from build123d import *

# Parameters (mm, degrees)
SKETCH1_R                    = 18.4
BOSS_EXTRUDE1_DEPTH          = 26.5
SKETCH2_R                    = 17.4
BOSS_EXTRUDE2_DEPTH          = 31
SKETCH3_R                    = 6
BOSS_EXTRUDE3_DEPTH          = 6.5
FILLET1_R                    = 0.5
SKETCH4_R                    = 3
BOSS_EXTRUDE4_DEPTH          = 15.5
CUT_EXTRUDE1_START           = -12
CUT_EXTRUDE1_DEPTH           = 12
F_3_0_3_DIAMETER_HOLE1_D     = 3
F_3_0_3_DIAMETER_HOLE1_DEPTH = 3
F_3_0_3_DIAMETER_HOLE1_TIP   = 0.901290929
CUT_EXTRUDE2_DEPTH           = 1
SKETCH9_R                    = 4
BOSS_EXTRUDE5_DEPTH          = 1
FILLET2_R                    = 0.5
SKETCH10_R                   = 14
BOSS_EXTRUDE6_DEPTH          = 1.5
SKETCH11_W                   = 3.5
SKETCH11_H                   = 1
BOSS_EXTRUDE7_DEPTH          = 5.6
FILLET3_R                    = 0.5
SKETCH13_R                   = 9
BOSS_EXTRUDE8_DEPTH          = 3
SKETCH14_R                   = 1.5
BOSS_EXTRUDE9_DEPTH          = 8.55
FILLET4_R                    = 0.5
SKETCH15_R                   = 16.4
BOSS_EXTRUDE10_DEPTH         = 15.26


with BuildPart() as part:
    # Sketch1 → Boss-Extrude1 (new body)
    with BuildSketch(Plane.XY):
        Circle(SKETCH1_R)
    extrude(amount=BOSS_EXTRUDE1_DEPTH)

    # Sketch2 → Boss-Extrude2 (add)
    with BuildSketch(Plane(origin=(0, 0, 0), x_dir=(-1, 0, 0), z_dir=(0, 0, -1))):
        with Locations(Location((0, 0, 0), (0, 0, 180))):
            Circle(SKETCH2_R)
    extrude(amount=BOSS_EXTRUDE2_DEPTH)

    # Sketch3 → Boss-Extrude3 (add)
    with BuildSketch(Plane.XY.offset(26.5)):
        with Locations(Location((7, 0, 0), (0, 0, 180))):
            Circle(SKETCH3_R)
    extrude(amount=BOSS_EXTRUDE3_DEPTH)

    # Fillet1
    fillet1_edges = [part.edges().sort_by_distance(p)[0] for p in [
        (13, 0, 33),
    ]]
    fillet(fillet1_edges, radius=FILLET1_R)

    # Sketch4 → Boss-Extrude4 (add)
    with BuildSketch(Plane.XY.offset(33)):
        with Locations((7, 0)):
            Circle(SKETCH4_R)
    extrude(amount=BOSS_EXTRUDE4_DEPTH)

    # Sketch5 → Cut-Extrude1 (cut)
    with BuildSketch(Plane.XY.offset(48.5).offset(CUT_EXTRUDE1_START)):
        with BuildLine():
            Line((5.503337045, 2.6), (8.496662955, 2.6))
            ThreePointArc((8.496662955, 2.6), (7, 3), (5.503337045, 2.6))
        make_face()
    extrude(amount=CUT_EXTRUDE1_DEPTH, mode=Mode.SUBTRACT)

    # Ø3.0 (3) Diameter Hole1
    with Locations(Plane.XY.offset(26.5)):
        with Locations((-13.423393759, 7.75), (-13.423393759, -7.75), (0, -15.5), (13.423393759, 7.75), (0, 15.5), (13.423393759, -7.75)):
            Hole(F_3_0_3_DIAMETER_HOLE1_D / 2, depth=F_3_0_3_DIAMETER_HOLE1_DEPTH)
            with Locations((0, 0, -(F_3_0_3_DIAMETER_HOLE1_DEPTH + F_3_0_3_DIAMETER_HOLE1_TIP / 2))):  # 118° drill point
                Cone(0, F_3_0_3_DIAMETER_HOLE1_D / 2, F_3_0_3_DIAMETER_HOLE1_TIP, mode=Mode.SUBTRACT)

    # Sketch8 → Cut-Extrude2 (cut)
    with BuildSketch(Plane.XY.offset(26.5)):
        with BuildLine():
            ThreePointArc((10.116155685, 7.342574083), (-12.5, 0), (10.116155685, -7.342574083))
            ThreePointArc((10.116155685, -7.342574083), (-1.05978604, 0), (10.116155685, 7.342574083))
        make_face()
    extrude(amount=-CUT_EXTRUDE2_DEPTH, mode=Mode.SUBTRACT)

    # Sketch9 → Boss-Extrude5 (add)
    with BuildSketch(Plane(origin=(0, 0, -31), x_dir=(-1, 0, 0), z_dir=(0, 0, -1))):
        Circle(SKETCH9_R)
    extrude(amount=BOSS_EXTRUDE5_DEPTH)

    # Fillet2
    fillet2_edges = [part.edges().sort_by_distance(p)[0] for p in [
        (4, 0, -32),
    ]]
    fillet(fillet2_edges, radius=FILLET2_R)

    # Sketch11 → Boss-Extrude7 (add)
    with BuildSketch(Plane(origin=(0, 0, -31), x_dir=(-1, 0, 0), z_dir=(0, 0, -1))):
        with Locations((0, 12.05)):
            Rectangle(SKETCH11_W, SKETCH11_H)
        with Locations((0, -12.05)):
            Rectangle(SKETCH11_W, SKETCH11_H)
    extrude(amount=BOSS_EXTRUDE7_DEPTH)

    # Fillet3
    fillet3_edges = [part.edges().sort_by_distance(p)[0] for p in [
        (1.75, 12.05, -36.6),
        (-1.75, 12.05, -36.6),
        (-1.75, -12.05, -36.6),
        (1.75, -12.05, -36.6),
    ]]
    fillet(fillet3_edges, radius=FILLET3_R)

    # Sketch14 → Boss-Extrude9 (add)
    with BuildSketch(Plane(origin=(0, 0, -32), x_dir=(-1, 0, 0), z_dir=(0, 0, -1))):
        Circle(SKETCH14_R)
    extrude(amount=BOSS_EXTRUDE9_DEPTH)

    # Fillet4
    # the kernel refuses this fillet: 0.5 mm, written as the material it takes off along each edge
    with BuildSketch(Plane(origin=(7, 0, 48.5), x_dir=(0.4622655728594592, 0.8867415295050277, 0), z_dir=(0.8867415295050277, -0.4622655728594592, 0))) as fillet4_piece_1:
        with BuildLine():
            CenterArc((3 - FILLET4_R, -FILLET4_R), FILLET4_R, 0, 90)
            Line((3 - FILLET4_R, 0), (3 - FILLET4_R, FILLET4_R * 0.02))
            Line((3 - FILLET4_R, FILLET4_R * 0.02), (3 + FILLET4_R * 0.02, FILLET4_R * 0.02))
            Line((3 + FILLET4_R * 0.02, FILLET4_R * 0.02), (3 + FILLET4_R * 0.02, -FILLET4_R))
            Line((3 + FILLET4_R * 0.02, -FILLET4_R), (3, -FILLET4_R))
        make_face()
    revolve(axis=Axis((7, 0, 48.5), (0, 0, 1)), revolution_arc=297.533397677, mode=Mode.SUBTRACT)
    with BuildSketch(Plane(origin=(7, 0, 48.5), x_dir=(1, 0, 0), z_dir=(0, -1, 0))) as fillet4_piece_2:
        with BuildLine():
            CenterArc((3 - FILLET4_R, -FILLET4_R), FILLET4_R, 0, 90)
            Line((3 - FILLET4_R, 0), (3 - FILLET4_R, FILLET4_R * 0.02))
            Line((3 - FILLET4_R, FILLET4_R * 0.02), (3 + FILLET4_R * 0.02, FILLET4_R * 0.02))
            Line((3 + FILLET4_R * 0.02, FILLET4_R * 0.02), (3 + FILLET4_R * 0.02, -FILLET4_R))
            Line((3 + FILLET4_R * 0.02, -FILLET4_R), (3, -FILLET4_R))
        make_face()
    revolve(axis=Axis((7, 0, 48.5), (0, 0, 1)), revolution_arc=117.379597562, mode=Mode.SUBTRACT)



with BuildPart() as body_2:
    # Sketch10 → Boss-Extrude6 (new body)
    with BuildSketch(Plane(origin=(0, 0, -34), x_dir=(-1, 0, 0), z_dir=(0, 0, -1))):
        Circle(SKETCH10_R)
    extrude(amount=BOSS_EXTRUDE6_DEPTH)


with BuildPart() as body_3:
    # Sketch13 → Boss-Extrude8 (new body)
    with BuildSketch(Plane(origin=(0, 0, -37.5), x_dir=(-1, 0, 0), z_dir=(0, 0, -1))):
        Circle(SKETCH13_R)
    extrude(amount=BOSS_EXTRUDE8_DEPTH)


with BuildPart() as part_1:
    add(part.part)

    add(body_2.part)  # Boss-Extrude10 merges body 2

    add(body_3.part)  # Boss-Extrude10 merges body 3
    # Sketch15 → Boss-Extrude10 (add)
    with BuildSketch(Plane(origin=(0, 0, -31), x_dir=(-1, 0, 0), z_dir=(0, 0, -1))):
        Circle(SKETCH15_R)
    extrude(amount=BOSS_EXTRUDE10_DEPTH)


solid = part_1.part
The listing builds one solid part. Answer for the finished solid, in the listing's coordinates (mm). A direction names the side the tool comes from. Coordinates: 2 decimals unless noted, no trailing zeros. Order: outer loops, then holes, each group sorted by start corner. A loop starts at its lowest first (then second) coordinate and runs counter-clockwise, first axis right, second up.
Q1. Consider line 1 (X direction, y = -7.75, z = 24.6); line 2 (Z direction, x = 2, y = 10); line 3 (X direction, y = 15.5, z = 25.15). Determine where each line is inside the solid, lowest interval first.
Q2. A cutting plane is placed at C-C, the plane x = -4. Write down the section's boundary in (y, z).
Q3. A cutting plane is placed at A-A, the plane z = 24.5. Write down the section's boundary in (x, y), and give its area (3 significant figures).
Q4. A cutting plane is placed at D-D, the plane z = -26. Write down the section's boundary in (x, y).
Q5. Given P1, Ø3.5, axis at x = 7.5, z = 39.5, coming from the +Y side; P2, Ø5, axis at x = 14, y = -3.5, coming from the +Z side; P3, Ø4, axis at x = 13.42, y = 7.75, coming from the +Z side, each flat-ended and moving along its own axis, determine where each tip first touches the part or whether it passes through.
Q6. Which of the six approach directions +Z, -Z, +X, -X, +Y, -Y give full straight-line access (tool end or side, diameter ignored) to faces 1 (the face through (0, -17, 25)), 2 (the face through (7, 0, 48.5)), 3 (the face through (14, 11, 0))?
Q7. For a pull along Y with two mould halves and no side action, classify faces 4 (the face through (13.544, -7.981, 22.755)), 5 (the face through (7, 2.6, 42)), 6 (the face through (0, 0, -46.26)) as pulls with the +Y half, pulls with the -Y half, needs draft (parallel to the pull), parting line crosses it, or undercut.
Q8. A cutting plane is placed at B-B, the plane y = 0. Write down the section's boundary in (x, z).
Answers follow:
1. line 1: x = -16.69 to -14.92, -11.92 to 11.92, 14.92 to 16.69
1. line 2: z = -46.26 to 25.5
1. line 3: x = -9.92 to -1.5, 1.5 to 9.92
2. outline: (-17.96, 0) - (-16.93, 0) - (-16.93, -31) - (-15.9, -31) - (-15.9, -46.26) - (15.9, -46.26) - (15.9, -31) - (16.93, -31) - (16.93, 0) - (17.96, 0) - (17.96, 26.5) - (11.84, 26.5) - (11.84, 25.5) - (-11.84, 25.5) - (-11.84, 26.5) - (-17.96, 26.5) - close
3. outline: circle Ø36.8 at (0, 0); hole circle Ø3 at (-13.42, -7.75); hole circle Ø3 at (-13.42, 7.75); hole circle Ø3 at (0, -15.5); hole circle Ø3 at (0, 15.5); hole circle Ø3 at (13.42, -7.75); hole circle Ø3 at (13.42, 7.75)
3. area: 1,020 mm2
4. outline: circle Ø34.8 at (0, 0)
5. P1: stops at y = 2.6
5. P2: stops at z = 33
5. P3: stops at z = 26.5
6. face 1: +Z
6. face 2: +Z, +X, -X, +Y, -Y
6. face 3: -Z
7. face 4: undercut
7. face 5: pulls with the +Y half
7. face 6: needs draft
8. outline: (-18.4, 0) - (-17.4, 0) - (-17.4, -31) - (-16.4, -31) - (-16.4, -46.26) - (16.4, -46.26) - (16.4, -31) - (17.4, -31) - (17.4, 0) - (18.4, 0) - (18.4, 26.5) - (13, 26.5) - (13, 32.5) arc R0.5 ccw to (12.5, 33) - (10, 33) - (10, 48) arc R0.5 ccw to (9.5, 48.5) - (4.5, 48.5) arc R0.5 ccw to (4, 48) - (4, 33) - (1.5, 33) arc R0.5 ccw to (1, 32.5) - (1, 26.5) - (-1.06, 26.5) - (-1.06, 25.5) - (-12.5, 25.5) - (-12.5, 26.5) - (-18.4, 26.5) - close
